```python
from build123d import *

# Parameters (mm, degrees)
F0_W     = 20
F0_H     = 80
F1_DEPTH = 2
F2_DEPTH = 10


with BuildPart() as f1:
    # F0 (on Top) → F1 (new body)
    with BuildSketch(Plane.XY):
        Rectangle(F0_W, F0_H)
        Polygon((-10, -40), (-10, 40), (-11, 35.101021), (-11, -28.898979), align=None)
        Polygon((11, 35.101021), (10, 40), (10, -40), (11, -28.898979), align=None)
        Polygon((-11, -28.898979), (-11, 35.101021), (-15, 15.505103), align=None)
        Polygon((15, 15.505103), (11, 35.101021), (11, -28.898979), align=None)
    extrude(amount=F1_DEPTH)

    # F0 (on Top) → F2 (join)
    with BuildSketch(Plane.XY):
        Polygon((-15, 15.505103), (-11, 35.101021), (-11, 41), (-16.125, 15.89273), (-11, -41), (-11, -28.898979), align=None)
        Polygon((-10, 40), (10, 40), (11, 35.101021), (11, 41), (-11, 41), (-11, 35.101021), align=None)
        Polygon((11, 41), (11, 35.101021), (15, 15.505103), (11, -28.898979), (11, -41), (16.125, 15.89273), align=None)
        Polygon((11, -28.898979), (10, -40), (-10, -40), (-11, -28.898979), (-11, -41), (11, -41), align=None)
    extrude(amount=F2_DEPTH)


solid = f1.part
```
Verification items for the finished model (mm, model axes). A direction names the side the tool comes from. Coordinates: 2 decimals unless noted, no trailing zeros. Loops run counter-clockwise (first coordinate to the right, second up) from the corner with the lowest first, then second, coordinate; pieces in that order, holes last. Notation, with made-up numbers: (34, -21.5) - (80, -21.5) arc R17 cw to (80, -2.5) - close; hole circle Ø3 at (-22, 33.25). An arc over 180 degrees is marked (long way). Put each result on its own line as item: value.
Item 1: Section check A-A (z = 3.25). Enter the section's corners in (x, y) (3 decimals), then the cut area to 3 significant figures.
Conclusion:
outline: (-16.125, 15.893) - (-11, -41) - (11, -41) - (16.125, 15.893) - (11, 41) - (-11, 41) - close; hole (-15, 15.505) - (-10, -40) - (10, -40) - (15, 15.505) - (10, 40) - (-10, 40) - close
area: 224 mm2
Item 2: Scan lines: line 1 along Y through (x, z) = (-2, 5); line 2 along Z through (x, y) = (6, 33.5); line 3 along X through (y, z) = (19, 3.5). Record each from-to range of solid material in increasing order.
Conclusion:
line 1: y = -41 to -40, 40 to 41
line 2: z = 0 to 2
line 3: x = -15.49 to -14.29, 14.29 to 15.49
Item 3: Draft check along Y on faces 1 (the face through (0, 1, 2)), 2 (the face through (0, -41, 5)), 3 (the face through (13.6, 28.27, 4.93)). Enter one of: pulls with the +Y half, pulls with the -Y half, needs draft (parallel to the pull), parting line crosses it, or undercut.
Conclusion:
face 1: undercut
face 2: pulls with the -Y half
face 3: pulls with the +Y half
Item 4: Gauge pin test, flat ends, axial feed: pin 1 Ø8 at (x, y) = (-3, 27.5) entering from -Z; pin 2 Ø6 at (y, z) = (4.5, 4.5) entering from +X; pin 3 Ø4 at (y, z) = (19, 3.5) entering from -X; pin 4 Ø12 at (x, y) = (2.5, 27.5) entering from +Z. Record the tip position at first contact, or that the pin passes through.
Conclusion:
pin 1: stops at z = 0
pin 2: stops at x = 15.37
pin 3: stops at x = -15.9
pin 4: stops at z = 2
Item 5: Section check B-B (x = -1). Enter the section's corners in (y, z), then the cut area to 3 significant figures.
Conclusion:
outline: (-41, 0) - (41, 0) - (41, 10) - (40, 10) - (40, 2) - (-40, 2) - (-40, 10) - (-41, 10) - close
area: 180 mm2
Item 6: Set-up check for faces 4 (the face through (-13.598, -12.155, 4.93)), 5 (the face through (0, 40, 6)): record each of +Z, -Z, +X, -X, +Y, -Y from which the full face is reachable in a straight line by a thin tool's end or side.
Conclusion:
face 4: +Z, -Z, -X, -Y
face 5: +Z
Item 7: Section check C-C (y = -20). Enter the section's corners in (x, z), then the cut area to 3 significant figures.
Conclusion:
outline: (-12.89, 0) - (12.89, 0) - (12.89, 10) - (11.8, 10) - (11.8, 2) - (-11.8, 2) - (-11.8, 10) - (-12.89, 10) - close
area: 69.0 mm2
